For this review, use the dimensioned drawing (mm, ordinates from the lowest corner) and the shaded views. A direction names the side the tool comes from. Give positions to 0.01 mm unless a question says otherwise; leave off trailing zeros. Write each loop counter-clockwise with the first axis right and the second up, starting at its lowest first coordinate (ties: lowest second). Pieces come first, ordered by that corner, then holes. Notation, with made-up numbers: (28, -26) -> (50, -26) arc R28 cw to (50, 3) -> close; hole circle Ø10 at (0, 11.5). An arc over 180 degrees is marked (long way). Write each question's results on one line, items separated by ' | '. Start each with the question number.
(1) Take a section at A-A (x = 175). State the section outline as (y, z) points.
(2) To check wall thickness, follow probe 1 along Z at (x, y) = (300.5, 184.5); probe 2 along X at (y, z) = (176.5, 68); probe 3 along Y at (x, z) = (230.5, 129). State the ranges of each line that lie inside material, in increasing order.
(3) Clearance check with flat-ended pins moving along their axes: pin 1 (12 mm diameter, centred on x = 134.5, z = 134.5, fed in from -Y); pin 2 (1.5 mm diameter, centred on x = 177.5, z = 24.5, fed in from -Y); pin 3 (8 mm diameter, centred on x = 56, z = 93.5, fed in from +Y). State where each tip first meets the part, or that it passes through.
(4) Take a section at C-C (z = 55). State the section outline as (x, y) points.
(5) Take a section at D-D (x = 215). State the section outline as (y, z) points.
(6) For the marked faces 1 and 2, list the 3-axis set-ups (+Z, -Z, +X, -X, +Y, -Y) from which the entire face can be reached by the end or side of a thin tool; tool diameter is ignored.
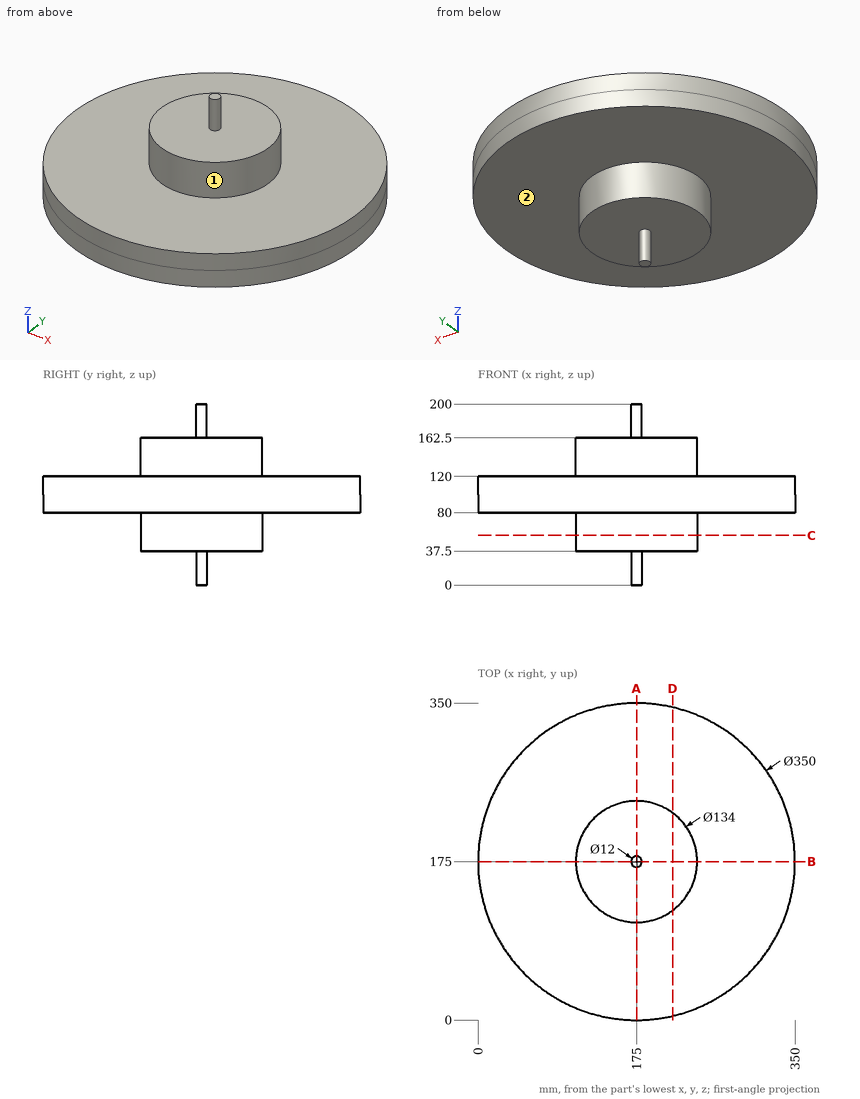
Report:
1) outline: (0, 80) -> (108, 80) -> (108, 37.5) -> (169, 37.5) -> (169, 0) -> (181, 0) -> (181, 37.5) -> (242, 37.5) -> (242, 80) -> (350, 80) -> (350, 120) -> (242, 120) -> (242, 162.5) -> (181, 162.5) -> (181, 200) -> (169, 200) -> (169, 162.5) -> (108, 162.5) -> (108, 120) -> (0, 120) -> close
2) probe 1: 80 to 120 | probe 2: 108.02 to 241.98 | probe 3: 137.47 to 212.53
3) pin 1: y = 117.57 | pin 2: y = 169.26 | pin 3: y = 306.91
4) outline: circle Ø134 at (175, 175)
5) outline: (4.63, 80) -> (121.25, 80) -> (121.25, 37.5) -> (228.75, 37.5) -> (228.75, 80) -> (345.37, 80) -> (345.37, 120) -> (228.75, 120) -> (228.75, 162.5) -> (121.25, 162.5) -> (121.25, 120) -> (4.63, 120) -> close
6) face 1: +Z | face 2: -Z
